Geometry: final body of the model. Coordinates: model frame, mm. Face numbers are marked on the shaded views. A direction names the side the tool comes from. Give positions to 0.01 mm unless a question says otherwise; leave off trailing zeros. Write each loop counter-clockwise with the first axis right and the second up, starting at its lowest first coordinate (ties: lowest second). Pieces come first, ordered by that corner, then holes. Notation, with made-up numbers: (6, -32) -> (24, -32) arc R7 cw to (24, -21) -> close; hole circle Ø3 at (13, 13.25). An arc over 180 degrees is marked (long way). Use CSV: the item, a comma, the result in double quotes. Start each with the question number.
1) Section D-D (x = -19). Output: boundary loops of the cut face in (y, z).
2) Draft query along Z for the marked faces 1, 2 and 3. Return one class per face: pulls with the +Z half, pulls with the -Z half, needs draft (parallel to the pull), parting line crosses it, or undercut.
3) Section A-A (x = 0). Output: boundary loops of the cut face in (y, z).
4) Material intervals for line 1 (Z direction, x = 0, y = 1); line 2 (Z direction, x = 0, y = 12); line 3 (Y direction, x = 50.5, z = 11.5), sorted ascending. Write a range as [from, to].
5) Section B-B (z = -11.5). Output: boundary loops of the cut face in (x, y), plus the area to 3 significant figures.
6) Set-up query: the marked faces 4 and 5. Return all of +Z, -Z, +X, -X, +Y, -Y with unobstructed straight access to the full face (end or side cutting, diameter ignored); none if empty.
7) Section C-C (y = 45.5). Output: boundary loops of the cut face in (x, z).
8) Contact query for a flat-ended pin moving along its axis: P1, Ø8, axis at x = -50.5, z = -40.5, coming from the +Y side. Output: stop coordinate, or through.
```python
from build123d import *

# Parameters (mm, degrees)
SKETCH_1_W      = 160
SKETCH_1_H      = 160
EXTRUDE_1_DEPTH = 60


with BuildPart() as part:
    # 草圖1 → 填料-伸長1 (new body)
    with BuildSketch(Plane(origin=(0, 0, 0), x_dir=(1, 0, 0), z_dir=(0, 1, 0))):
        Rectangle(SKETCH_1_W, SKETCH_1_H)
    extrude(amount=EXTRUDE_1_DEPTH)

    # 草圖2 → 除料-旋轉1 (revolve, cut)
    with BuildSketch(Plane.XY):
        Polygon((0, 0), (14, 0), (14, 5), (50, 5), (50, 15), (60, 15), (60, 17), (70, 17), (70, 60), (0, 60), align=None)
    revolve(axis=Axis((0, 77.889426339, 0), (0, -1, 0)), mode=Mode.SUBTRACT)


solid = part.part
```
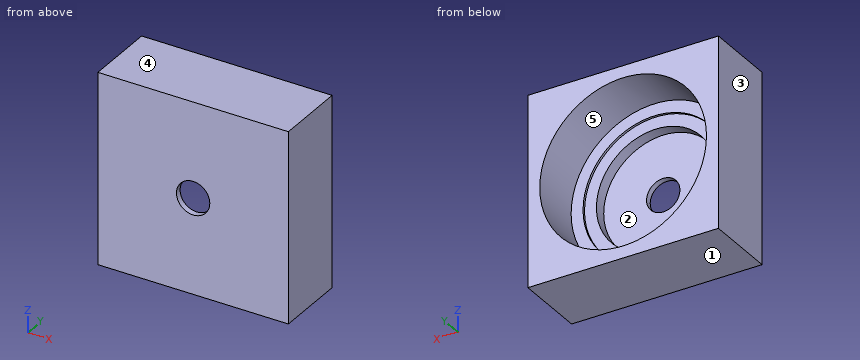
Answers follow:
1,outline,"(0, -80) -> (60, -80) -> (60, -67.37) -> (17, -67.37) -> (17, -56.91) -> (15, -56.91) -> (15, -46.25) -> (5, -46.25) -> (5, 46.25) -> (15, 46.25) -> (15, 56.91) -> (17, 56.91) -> (17, 67.37) -> (60, 67.37) -> (60, 80) -> (0, 80) -> close"
2,face 1,"pulls with the -Z half"
2,face 2,"undercut"
2,face 3,"needs draft"
3,outline,"(0, -80) -> (60, -80) -> (60, -70) -> (17, -70) -> (17, -60) -> (15, -60) -> (15, -50) -> (5, -50) -> (5, -14) -> (0, -14) -> close; (0, 14) -> (5, 14) -> (5, 50) -> (15, 50) -> (15, 60) -> (17, 60) -> (17, 70) -> (60, 70) -> (60, 80) -> (0, 80) -> close"
4,line 1,"z = [-80, -14], [14, 80]"
4,line 2,"z = [-80, -50], [50, 80]"
4,line 3,"y = [0, 15]"
5,outline,"(-80, 0) -> (-7.98, 0) -> (-7.98, 5) -> (-48.66, 5) -> (-48.66, 15) -> (-58.89, 15) -> (-58.89, 17) -> (-69.05, 17) -> (-69.05, 60) -> (-80, 60) -> close; (7.98, 0) -> (80, 0) -> (80, 60) -> (69.05, 60) -> (69.05, 17) -> (58.89, 17) -> (58.89, 15) -> (48.66, 15) -> (48.66, 5) -> (7.98, 5) -> close"
5,area,"2,370 mm^2"
6,face 4,"+Z, +X, -X, +Y, -Y"
6,face 5,"+Y"
7,outline,"(-80, -80) -> (80, -80) -> (80, 80) -> (-80, 80) -> close; hole circle Ø140 at (0, 0)"
8,P1,"stops at y = 17"
